Design review of the part built by this model. Coordinates are the model's own, in mm. Coordinates: 2 decimals unless noted, no trailing zeros. Write each loop counter-clockwise with the first axis right and the second up, starting at its lowest first coordinate (ties: lowest second). Pieces come first, ordered by that corner, then holes.
```python
from build123d import *

# Parameters (mm, degrees)
F0_W     = 400
F0_H     = 30
F1_ANGLE = 10
F4_D     = 6
F4_DEPTH = 100


with BuildPart() as f1:
    # F0 (on Right) → F1 (revolve, symmetric)
    with BuildSketch(Plane.YZ) as f1_sk:
        with Locations((0, 1569)):
            Rectangle(F0_W, F0_H)
    revolve(axis=Axis((0, -0.207613, 0), (0, 1, 0)), revolution_arc=F1_ANGLE / 2)
    revolve(f1_sk.sketch, axis=Axis((0, -0.207613, 0), (0, -1, 0)), revolution_arc=F1_ANGLE / 2)

    # F4
    with Locations(Plane.XY.offset(1600)):
        with Locations((-113.054697, 175), (113.054697, -175)):
            Hole(F4_D / 2, depth=F4_DEPTH)


solid = f1.part
```
(1) Mouldability with a two-part tool opening along X and no side actions: class faces 1 (the flat face through (-2, 200, 1566)), 2 (the cylindrical face through (2, 3, 1554)), 3 (the cylindrical face through (2, 3, 1584)) as +X half, -X half, draft (parallel to the pull), parting line (faces both ways), or undercut.
(2) Wall thickness on line 1 (Y direction, x = -112.5, z = 1553.5); line 2 (X direction, y = -175, z = 1574); line 3 (X direction, y = -175, z = 1559): over which ranges is each line inside the solid? List them lowest first.
(3) Consider section B-B (x = 53). Give the boundary of the cut face in (y, z), plus the area to 3 significant figures.
(4) Consider section A-A (y = -49). Give the boundary of the cut face in (x, z).
(5) Insertion check: pin 1 Ø8 at (x, y) = (-113.05, 175) entering from -Z; pin 2 Ø1 at (y, z) = (-31.5, 1571.5) entering from +X; pin 3 Ø3 at (x, y) = (-99.5, 8) entering from -Z. Each pin has a flat end and moves straight along its axis. Give the tip position at first contact, or say it passes through.
Results:
1. face 1: draft
1. face 2: undercut
1. face 3: parting line
2. line 1: y = -200 to 172.05, 177.95 to 200
2. line 2: x = -137.71 to 110.05, 116.05 to 137.71
2. line 3: x = -136.39 to 110.05, 116.05 to 136.39
3. outline: (-200, 1553.1) - (200, 1553.1) - (200, 1583.11) - (-200, 1583.11) - close
3. area: 12,000 mm2
4. outline: (-138.05, 1577.97) - (-135.44, 1548.09) arc R1554 cw to (135.44, 1548.09) - (138.05, 1577.97) arc R1584 ccw to start
5. pin 1: stops at z = 1549.59
5. pin 2: stops at x = 137.53
5. pin 3: stops at z = 1550.71
